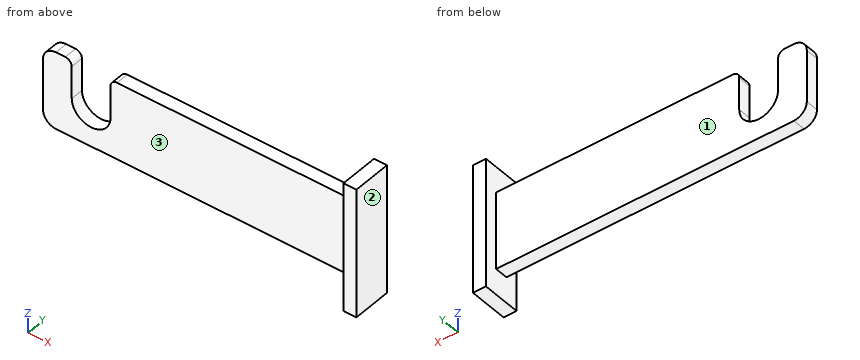
```python
from build123d import *

# Parameters (mm, degrees)
F1_DEPTH = 12.7
F2_W     = 38.1
F2_H     = 127
F3_DEPTH = 12.7


with BuildPart() as f1:
    # F0 (on Front) → F1 (new body)
    with BuildSketch(Plane.XZ):
        with BuildLine():
            Line((-139.7, -38.1), (152.4, -38.1))
            Line((152.4, -38.1), (152.4, 38.1))
            Line((152.4, 38.1), (-79.751387, 38.1))
            ThreePointArc((-79.751387, 38.1), (-84.241515, 36.240128), (-86.101387, 31.75))
            Line((-86.101387, 31.75), (-86.101387, 0))
            ThreePointArc((-86.101387, 0), (-105.151387, -19.05), (-124.201387, 0))
            Line((-124.201387, 0), (-124.201387, 31.75))
            ThreePointArc((-124.201387, 31.75), (-126.061259, 36.240128), (-130.551387, 38.1))
            Line((-130.551387, 38.1), (-139.7, 38.1))
            ThreePointArc((-139.7, 38.1), (-148.680256, 34.380256), (-152.4, 25.4))
            Line((-152.4, 25.4), (-152.4, -25.4))
            ThreePointArc((-152.4, -25.4), (-148.680256, -34.380256), (-139.7, -38.1))
        make_face()
    extrude(amount=F1_DEPTH)

    # F2 (on face) → F3 (join)
    with BuildSketch(Plane.YZ.offset(152.4)):
        with Locations((-6.35, 0)):
            Rectangle(F2_W, F2_H)
    extrude(amount=F3_DEPTH)


solid = f1.part
```
Geometry check sheet. Reference: the model listing, model coordinates, mm. Face numbers are marked on the shaded views. A direction names the side the tool comes from. Round coordinates to 2 decimals unless told otherwise and drop trailing zeros. Loops run counter-clockwise (first coordinate to the right, second up) from the corner with the lowest first, then second, coordinate; pieces in that order, holes last. Notation, with made-up numbers: (57.25, 52) - (84.25, 52) arc R21 ccw to (84.25, 86) - close; hole circle Ø2 at (50, -14.5). An arc over 180 degrees is marked (long way). Write each question's results on one line, items separated by ' | '. Start each with the question number.
Q1. Access from +Z, -Z, +X, -X, +Y, -Y to the whole of each face (thin tool, end or side, straight path). Record for the marked faces 1, 2 and 3.
Q2. Cross-section at C-C on x = 38.5. Enter the section's corners in (y, z), and give its area (3 significant figures).
Q3. Thickness scan on line 1 (X direction, y = -1, z = 23.5); line 2 (X direction, y = -8, z = 48.5); line 3 (Y direction, x = 124, z = 35.5). Record the ranges inside material, lowest first. Write a range as [from, to].
Q4. Gauge pin test, flat ends, axial feed: P1, Ø14, axis at x = 82, y = -6, coming from the +Z side; P2, Ø1, axis at x = -54.5, y = -5, coming from the -Z side; P3, Ø12, axis at x = -27.5, z = 16.5, coming from the +Y side; P4, Ø12, axis at x = -100.5, z = -11, coming from the -Y side. Record the tip position at first contact, or that the pin passes through.
Q5. Cross-section at D-D on z = -14. Enter the section's corners in (x, y).
Q6. Cross-section at A-A on z = 11. Enter the section's corners in (x, y), and give its area (3 significant figures).
Q7. Cross-section at B-B on y = -9.5. Enter the section's corners in (x, z).
Answers below:
1) face 1: +Z, -Z, -X, +Y | face 2: +Z, -Z, +X, +Y, -Y | face 3: +Z, -Z, -X, -Y
2) outline: (-12.7, -38.1) - (0, -38.1) - (0, 38.1) - (-12.7, 38.1) - close | area: 968 mm²
3) line 1: x = [-152.4, -124.2], [-86.1, 165.1] | line 2: x = [152.4, 165.1] | line 3: y = [-12.7, 0]
4) P1: stops at z = 38.1 | P2: stops at z = -38.1 | P3: stops at y = 0 | P4: passes through
5) outline: (-152.4, -12.7) - (-118.07, -12.7) - (-118.07, 0) - (-152.4, 0) - close; (-92.23, -12.7) - (152.4, -12.7) - (152.4, -25.4) - (165.1, -25.4) - (165.1, 12.7) - (152.4, 12.7) - (152.4, 0) - (-92.23, 0) - close
6) outline: (-152.4, -12.7) - (-124.2, -12.7) - (-124.2, 0) - (-152.4, 0) - close; (-86.1, -12.7) - (152.4, -12.7) - (152.4, -25.4) - (165.1, -25.4) - (165.1, 12.7) - (152.4, 12.7) - (152.4, 0) - (-86.1, 0) - close | area: 3,870 mm²
7) outline: (-152.4, -25.4) arc R12.7 ccw to (-139.7, -38.1) - (152.4, -38.1) - (152.4, -63.5) - (165.1, -63.5) - (165.1, 63.5) - (152.4, 63.5) - (152.4, 38.1) - (-79.75, 38.1) arc R6.35 ccw to (-86.1, 31.75) - (-86.1, 0) arc R19.05 cw to (-124.2, 0) - (-124.2, 31.75) arc R6.35 ccw to (-130.55, 38.1) - (-139.7, 38.1) arc R12.7 ccw to (-152.4, 25.4) - close
